Build history of the part. All positions in model axes, mm. A direction names the side the tool comes from. Round coordinates to 2 decimals unless told otherwise and drop trailing zeros. Loops run counter-clockwise (first coordinate to the right, second up) from the corner with the lowest first, then second, coordinate; pieces in that order, holes last. Notation, with made-up numbers: M 30,-23.75 L 75,-23.75 A9 ccw 75,-6.75 Z; hole C 75,-5.5 d4. An arc over 180 degrees is marked long. Write each question's results on one line, items separated by ' | '. Start each with the question number.
```python
from build123d import *

# Parameters (mm, degrees)
F1_DEPTH = 100


with BuildPart() as f1:
    # F0 (on Top) → F1 (new body)
    with BuildSketch(Plane.XY):
        with BuildLine():
            Line((-300, 300), (-250, 300))
            Line((-250, 300), (250, 300))
            Line((250, 300), (300, 300))
            Line((300, 300), (300, 250))
            Line((300, 250), (300, -300))
            Line((300, -300), (461.55284, -300))
            Line((461.55284, -300), (461.55284, -274.148953))
            Line((461.55284, -274.148953), (509.881234, -165.601602))
            Line((509.881234, -165.601602), (533.194239, -55.922539))
            Line((533.194239, -55.922539), (533.158025, 56.207051))
            Line((533.158025, 56.207051), (509.808885, 165.885914))
            Line((509.808885, 165.885914), (464.157372, 268.30564))
            Line((464.157372, 268.30564), (390.063715, 370.175778))
            Line((390.063715, 370.175778), (315.191048, 437.507966))
            Line((315.191048, 437.507966), (218.040579, 493.50566))
            Line((218.040579, 493.50566), (111.367142, 528.071001))
            Line((111.367142, 528.071001), (-0.534983, 539.73091))
            Line((-0.534983, 539.73091), (-112.787019, 527.820755))
            Line((-112.787019, 527.820755), (-220.106861, 492.822908))
            Line((-220.106861, 492.822908), (-317.800291, 436.268358))
            Line((-317.800291, 436.268358), (-401.594268, 360.630946))
            Line((-401.594268, 360.630946), (-467.848829, 269.184572))
            Line((-467.848829, 269.184572), (-513.780329, 166.020735))
            Line((-513.780329, 166.020735), (-537.307359, 55.319745))
            Line((-537.307359, 55.319745), (-537.307359, -52.090053))
            Line((-537.307359, -52.090053), (-350, -52.090053))
            ThreePointArc((-350, -52.090053), (-314.644661, -37.445392), (-300, -2.090053))
            Line((-300, -2.090053), (-300, 250))
            Line((-300, 250), (-300, 300))
        make_face()
    extrude(amount=F1_DEPTH)


solid = f1.part
```
Item 1: Saw through at D-D, the plane x = -47. Give the cut face in (y, z).
Item 2: Tool access for faces 5 (the flat face through (165.451, 510.546, 49.3)), 6 (the flat face through (-4, 300, 49)): list every direction of +Z, -Z, +X, -X, +Y, -Y with a clear straight run to the whole face (end or side of a thin tool).
Item 3: Saw through at B-B, the plane z = 65.5. Give the cut face in (x, y), then the cut area to 3 significant figures.
Item 4: Drop flat-ended pins along their axis: pin 1 (8 mm diameter, centred on y = -144, z = 67.5, fed in from +X); pin 2 (12 mm diameter, centred on x = -202, z = 21, fed in from -Y); pin 3 (8 mm diameter, centred on x = -175.5, z = 48.5, fed in from +Y). Give the stop position or say it passes through.
Item 5: Drill centre lines: line 1 along X through (y, z) = (281, 4); line 2 along X through (y, z) = (-89.5, 13); line 3 along Y through (x, z) = (150, 88). Where is each one in solid material? Low to high. Write a range as [from, to].
Item 6: Saw through at A-A, the plane y = 16. Give the cut face in (x, z), then the cut area to 3 significant figures.
Item 7: Mould opens along X. For faces 1 (the flat face through (461.553, -287, 49)), 2 (the flat face through (-300, 147, 49)), 3 (the cylindrical face through (-315.036, -37.832, 49.3)), 4 (the flat face through (-55.88, 533.86, 49.3)) say: released by +X, released by -X, zero draft, split by the parting line, or undercut.
Item 8: Saw through at C-C, the plane y = 223.5. Give the cut face in (x, z).
Working result:
1) outline: M 300,0 L 534.8,0 L 534.8,100 L 300,100 Z
2) face 5: +Z, -Z, +X, +Y | face 6: +Z, -Z, -Y
3) outline: M -537.31,-52.09 L -350,-52.09 A50 ccw -300,-2.09 L -300,300 L 300,300 L 300,-300 L 461.55,-300 L 461.55,-274.15 L 509.88,-165.6 L 533.19,-55.92 L 533.16,56.21 L 509.81,165.89 L 464.16,268.31 L 390.06,370.18 L 315.19,437.51 L 218.04,493.51 L 111.37,528.07 L -0.53,539.73 L -112.79,527.82 L -220.11,492.82 L -317.8,436.27 L -401.59,360.63 L -467.85,269.18 L -513.78,166.02 L -537.31,55.32 Z | area: 346,000 mm²
4) pin 1: stops at x = 515.32 | pin 2: stops at y = 300 | pin 3: stops at y = 508.67
5) line 1: x = [-459.29, -300], [300, 454.92] | line 2: x = [300, 526.06] | line 3: y = [300, 515.55]
6) outline: M -537.31,0 L -300,0 L -300,100 L -537.31,100 Z; M 300,0 L 533.17,0 L 533.17,100 L 300,100 Z | area: 47,000 mm²
7) face 1: released by +X | face 2: undercut | face 3: undercut | face 4: released by -X
8) outline: M -488.19,0 L -300,0 L -300,100 L -488.19,100 Z; M 300,0 L 484.13,0 L 484.13,100 L 300,100 Z
